Geometry check sheet. Reference: the model listing, model coordinates, mm. Round coordinates to 2 decimals unless told otherwise and drop trailing zeros. Order: outer loops, then holes, each group sorted by start corner. A loop starts at its lowest first (then second) coordinate and runs counter-clockwise, first axis right, second up. Notation, with made-up numbers: (0, -34) - (30, -34) arc R21 cw to (30, 4) - close; hole circle Ø11 at (70, 47). An arc over 180 degrees is marked (long way). Write each question's results on one line, items separated by ' | '.
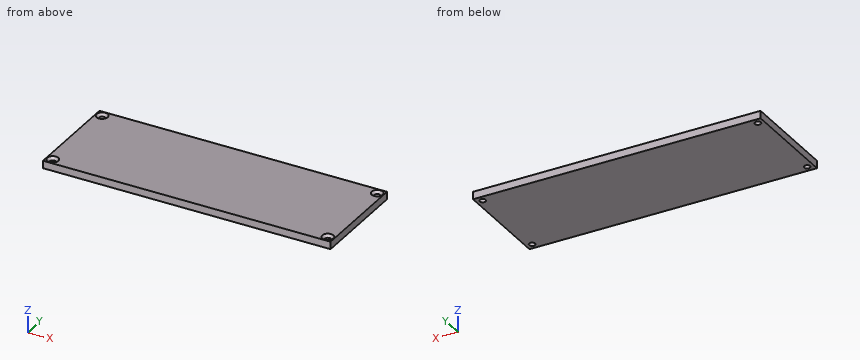
Autodesk Inventor part; units mm, degrees
ref_plane "YZ Plane" through (0, 0, 0) normal (1, 0, 0) x (0, 1, 0)
ref_plane "XZ Plane" through (0, 0, 0) normal (0, 1, 0) x (-1, 0, 0)
ref_plane "XY Plane" through (0, 0, 0) normal (0, 0, 1) x (1, 0, 0)
sketch "Skizze1" plane through (0, 0, 0) normal (0, 0, 1) x (1, 0, 0)
  line L0 (-23, 0) -> (138, 0)
  line L1 (0, -8) -> (0, 48)
  line L2 (0, 0) -> (115, 0)
  line L3 (115, 0) -> (115, 40)
  line L4 (115, 40) -> (0, 40)
  line L5 (0, 40) -> (0, 0)
  dimension "d0" = 40
  dimension "d1" = 115
extrude "Extrusion1" add sketch "Skizze1" along normal blind 3
sketch "Skizze2" plane through (0, 0, 3) normal (0, 0, 1) x (1, 0, 0)
  line L0 (0, 0) -> (115, 0)
  line L1 (115, 0) -> (115, 40)
  line L2 (115, 40) -> (0, 40)
  line L3 (0, 40) -> (0, 0)
  line L4 (2.5, 37.5) -> (112.5, 37.5)
  line L5 (112.5, 37.5) -> (112.5, 2.5)
  line L6 (112.5, 2.5) -> (2.5, 2.5)
  line L7 (2.5, 2.5) -> (2.5, 37.5)
  dimension "d5" = 2.5
hole "Bohrung1" at (2.5, 37.5, 3) at (2.5, 2.5, 3) at (112.5, 2.5, 3) at (112.5, 37.5, 3) direction (0, 0, -1) diameter 2.4 end through all countersink diameter 4.5 countersink angle 90
properties part number "13_1087_024"
(1) Section check A-A (y = 2.5). Record the cut outline in (x, z), then the cut area to 3 significant figures.
Answers follow:
outline: (0, 0) - (1.3, 0) - (1.3, 1.95) - (0.25, 3) - (0, 3) - close; (3.7, 0) - (111.3, 0) - (111.3, 1.95) - (110.25, 3) - (4.75, 3) - (3.7, 1.95) - close; (113.7, 0) - (115, 0) - (115, 3) - (114.75, 3) - (113.7, 1.95) - close | area: 328 mm²
(2) Material ranges on line 1 (Y direction, x = 112.5, z = 1.1); line 2 (X direction, y = 37.5, z = 0.7), recorded low to high.
Answers follow:
line 1: 0 to 1.3, 3.7 to 36.3, 38.7 to 40 | line 2: 0 to 1.3, 3.7 to 111.3, 113.7 to 115
(3) Section check B-B (x = 2.5). Record the cut outline in (y, z), then the cut area to 3 significant figures.
Answers follow:
outline: (0, 0) - (1.3, 0) - (1.3, 1.95) - (0.25, 3) - (0, 3) - close; (3.7, 0) - (36.3, 0) - (36.3, 1.95) - (35.25, 3) - (4.75, 3) - (3.7, 1.95) - close; (38.7, 0) - (40, 0) - (40, 3) - (39.75, 3) - (38.7, 1.95) - close | area: 103 mm²
